```python
from build123d import *

# Parameters (mm, degrees)
BOSS_EXTRUDE1_DEPTH    = 75
SKETCH9_R              = 11
BOSS_EXTRUDE3_DEPTH    = 25
BOSS_EXTRUDE4_DEPTH    = 6
F_12_0MM_DOWEL_HOLE1_D = 14


with BuildPart() as part:
    # Sketch1 → Boss-Extrude1 (new body)
    with BuildSketch(Plane.XY):
        Polygon((-16, -9), (-16, -3), (16, -3), (16, -9), (28, -9), (28, 9), (-28, 9), (-28, -9), align=None)
    extrude(amount=-BOSS_EXTRUDE1_DEPTH)



with BuildPart() as body_2:
    # Sketch9 → Boss-Extrude3 (new body)
    with BuildSketch(Plane(origin=(0, 54, 0), x_dir=(-1, 0, 0), z_dir=(0, -1, 0))):
        with BuildLine():
            Line((-55.029437252, 43.5), (-36, 43.5))
            Line((-36, 43.5), (-36, 31.5))
            Line((-36, 31.5), (-55.029437252, 31.5))
            ThreePointArc((-55.029437252, 31.5), (-90, 37.5), (-55.029437252, 43.5))
        make_face()
        with Locations(Location((-72, 37.5, 0), (0, 0, 180))):
            Circle(SKETCH9_R, mode=Mode.SUBTRACT)
    extrude(amount=BOSS_EXTRUDE3_DEPTH)


with BuildPart() as part_1:
    add(part.part)

    add(body_2.part)  # Boss-Extrude4 merges body 2
    # Sketch11 → Boss-Extrude4 (add, symmetric)
    with BuildSketch(Plane.XY.offset(-37.5)):
        Polygon((36, 29), (28, -9), (28, 9), (-28, 9), (36, 54), align=None)
    extrude(amount=BOSS_EXTRUDE4_DEPTH, both=True)

    # Ø12.0mm Dowel Hole1 (through all)
    with Locations(Plane(origin=(0, 9, 0), x_dir=(1, 0, 0), z_dir=(0, 1, 0))):
        with Locations((0, 15), (0, 60)):
            Hole(F_12_0MM_DOWEL_HOLE1_D / 2)


solid = part_1.part
```
Input: part model. Units: mm. Frame: model coordinates. A direction names the side the tool comes from. Round coordinates to 2 decimals unless told otherwise and drop trailing zeros. Loops run counter-clockwise (first coordinate to the right, second up) from the corner with the lowest first, then second, coordinate; pieces in that order, holes last.
1) Material intervals for line 1 (Z direction, x = 0, y = 5.75); line 2 (Z direction, x = 72, y = 46); line 3 (Y direction, x = 41, z = -37), sorted ascending.
Ans:
line 1: z = -75 to -67, -53 to -22, -8 to 0
line 2: z = -55.5 to -48.5, -26.5 to -19.5
line 3: y = 29 to 54
2) Set-up query: faces 4 (the flat face through (28, 0, -59)), 5 (the flat face through (0, 9, -52)), 6 (the flat face through (-16, -6, -37)). Return all of +Z, -Z, +X, -X, +Y, -Y with unobstructed straight access to the full face (end or side cutting, diameter ignored); none if empty.
Ans:
face 4: -Z, +X, +Y, -Y
face 5: -Z, +X, -X, +Y
face 6: +Z, -Z, -Y
3) Section query B-B on x = 75. Return the cut outline in (y, z), plus the area to 3 significant figures.
Ans:
outline: (29, -55.25) - (54, -55.25) - (54, -48.08) - (29, -48.08) - close; (29, -26.92) - (54, -26.92) - (54, -19.75) - (29, -19.75) - close
area: 358 mm2
4) Section query A-A on z = -15. Return the cut outline in (x, y), plus the area to 3 significant figures.
Ans:
outline: (-28, -9) - (-16, -9) - (-16, -3) - (-7, -3) - (-7, 9) - (-28, 9) - close; (7, -3) - (16, -3) - (16, -9) - (28, -9) - (28, 9) - (7, 9) - close
area: 648 mm2
5) Pin query (flat end, axial travel): pin 1 (1.8 mm diameter, centred on y = -5, z = -45.5, fed in from +X); pin 2 (19 mm diameter, centred on x = 28, y = 24, fed in from +Z); pin 3 (22.5 mm diameter, centred on x = 0, z = -15, fed in from -Y). Return the tip coordinate at first contact, or that it passes through.
Ans:
pin 1: stops at x = 28
pin 2: stops at z = -31.5
pin 3: stops at y = -3
6) Pull-direction query (X, two-part tool) for faces 1 (the flat face through (32, 10, -37)), 2 (the flat face through (3.552, 31.185, -37.416)), 3 (the cylindrical face through (0.91, 2.92, -66.94)); classes: released by +X, released by -X, zero draft, split by the parting line, or undercut.
Ans:
face 1: released by +X
face 2: released by -X
face 3: undercut
7) Section query C-C on y = -1.5. Return the cut outline in (x, z).
Ans:
outline: (-28, -75) - (28, -75) - (28, -43.5) - (29.58, -43.5) - (29.58, -31.5) - (28, -31.5) - (28, 0) - (-28, 0) - close; hole circle Ø14 at (0, -60); hole circle Ø14 at (0, -15)
8) Section query D-D on y = 49. Return the cut outline in (x, z).
Ans:
outline: (28.89, -43.5) - (55.03, -43.5) arc R18 ccw (long way) to (55.03, -31.5) - (28.89, -31.5) - close; hole circle Ø22 at (72, -37.5)
